Can you work these out from the drawing? Everything is in mm from the part's minimum corner. A direction names the side the tool comes from. Round coordinates to 2 decimals unless told otherwise and drop trailing zeros. Write each loop counter-clockwise with the first axis right and the second up, starting at its lowest first coordinate (ties: lowest second). Pieces come first, ordered by that corner, then holes. Notation, with made-up numbers: (41.5, 83.25) - (62.5, 83.25) arc R15 cw to (62.5, 90.25) - close; hole circle Ø9 at (17, 39). An arc over 180 degrees is marked (long way). One line per item, written item: value. Start each with the question number.
(1) If I drill on L1, parallel to Z at x = 100, y = 2.9; L2, parallel to Y at x = 19.5, z = 2.5; L3, parallel to Z at x = 134.5, y = 27, over which ranges is the centre line in solid material (lowest first)? Write a range as from..to.
(2) I want a section at B-B on y = 2. List the corners of the cut face in (x, z) for me, plus the area to 3 significant figures.
(3) I want a section at D-D on x = 98. List the corners of the cut face in (y, z) for me.
(4) I want a section at A-A on z = 22. List the corners of the cut face in (x, y) for me.
(5) On a 3-axis mill with a long thin cutter (end or side, diameter ignored), from which of +Z, -Z, +X, -X, +Y, -Y can I reach the whole of each face in a straight line? I mean the marked faces 1 and 2. Say none if no direction works.
(6) I'm going to push flat-ended pins straight in: pin 1 Ø4 at (x, y) = (49, 13.5) entering from -Z; pin 2 Ø8 at (x, z) = (50, 19) entering from -Y; pin 3 Ø1.5 at (x, z) = (119, 17) entering from +Y. Where does each tip first touch, or does it pass through?
(7) I want a section at C-C on x = 50. List the corners of the cut face in (y, z) for me.
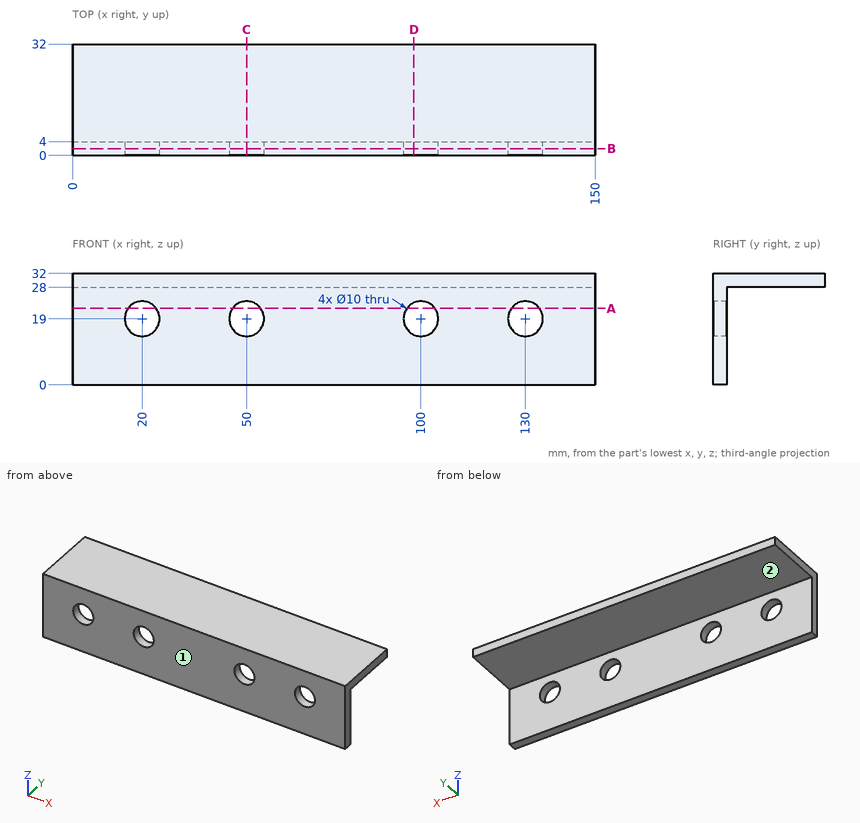
Established:
1. L1: 0..14, 24..32
1. L2: 0..4
1. L3: 28..32
2. outline: (0, 0) - (150, 0) - (150, 32) - (0, 32) - close; hole circle Ø10 at (20, 19); hole circle Ø10 at (50, 19); hole circle Ø10 at (100, 19); hole circle Ø10 at (130, 19)
2. area: 4,490 mm2
3. outline: (0, 0) - (4, 0) - (4, 14.42) - (0, 14.42) - close; (0, 23.58) - (4, 23.58) - (4, 28) - (32, 28) - (32, 32) - (0, 32) - close
4. outline: (0, 0) - (16, 0) - (16, 4) - (0, 4) - close; (24, 0) - (46, 0) - (46, 4) - (24, 4) - close; (54, 0) - (96, 0) - (96, 4) - (54, 4) - close; (104, 0) - (126, 0) - (126, 4) - (104, 4) - close; (134, 0) - (150, 0) - (150, 4) - (134, 4) - close
5. face 1: +Z, -Z, +X, -X, -Y
5. face 2: -Z, +X, -X, +Y
6. pin 1: z = 28
6. pin 2: through
6. pin 3: y = 4
7. outline: (0, 0) - (4, 0) - (4, 14) - (0, 14) - close; (0, 24) - (4, 24) - (4, 28) - (32, 28) - (32, 32) - (0, 32) - close
